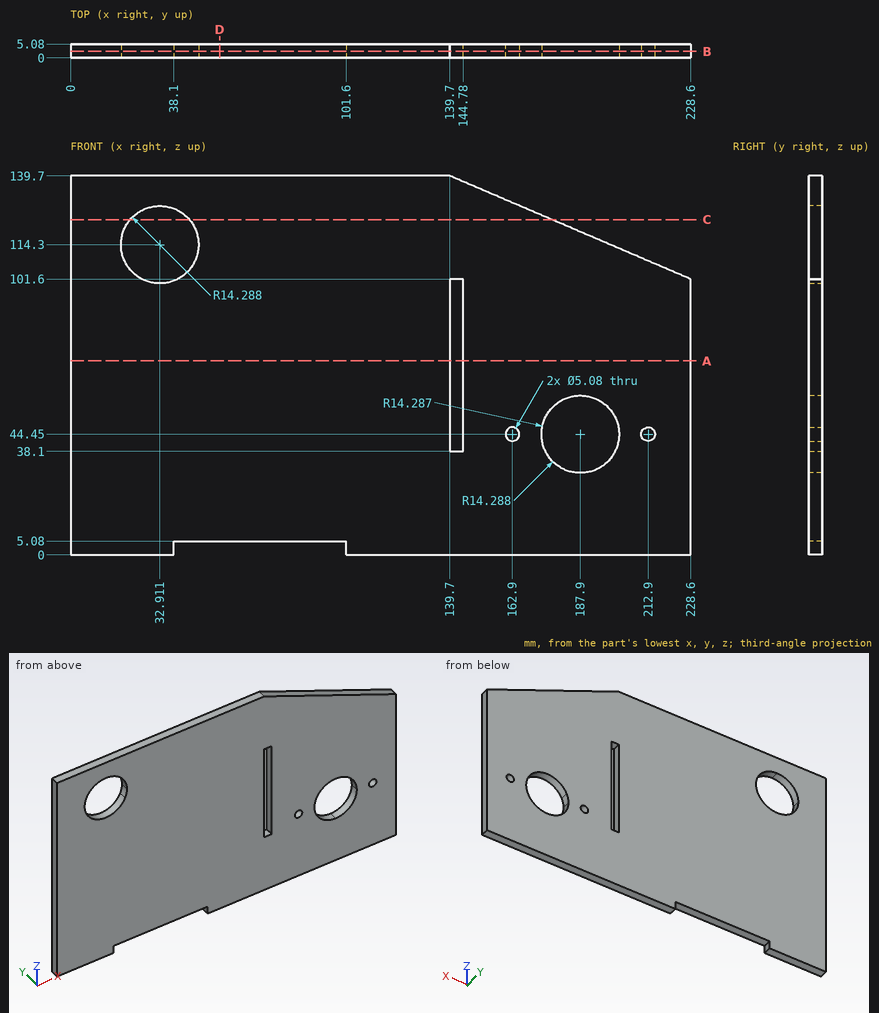
Part print with two shaded views. Sizes in mm from the minimum x, y, z corner. Give positions to 0.01 mm unless a question says otherwise; leave off trailing zeros. Order: outer loops, then holes, each group sorted by start corner. A loop starts at its lowest first (then second) coordinate and runs counter-clockwise, first axis right, second up.
1) Saw through at B-B, the plane y = 2.35. Count the separate pieces of the cut face and the enclosed holes in it, then the cut area to 3 significant figures.
2) Wall check: probe 1 along X at (y, z) = (4.45, 44.5); probe 2 along X at (y, z) = (0.3, 70); probe 3 along Z at (x, y) = (89, 4.55). Give the ranges that are in metal, low to high.
3) Saw through at A-A, the plane z = 71.5. Write the cut outline in (x, y).
4) Saw through at C-C, the plane z = 123.5. Write the cut outline in (x, y).
5) Saw through at D-D, the plane x = 55. Write the cut outline in (y, z).
Computed:
1. separate pieces: 1
1. enclosed holes: 5
1. area: 28,300 mm2
2. probe 1: x = 0 to 139.7, 144.78 to 160.36, 165.44 to 173.61, 202.19 to 210.36, 215.44 to 228.6
2. probe 2: x = 0 to 139.7, 144.78 to 228.6
2. probe 3: z = 5.08 to 139.7
3. outline: (0, 0) - (139.7, 0) - (139.7, 5.08) - (0, 5.08) - close; (144.78, 0) - (228.6, 0) - (228.6, 5.08) - (144.78, 5.08) - close
4. outline: (0, 0) - (21.98, 0) - (21.98, 5.08) - (0, 5.08) - close; (43.84, 0) - (177.5, 0) - (177.5, 5.08) - (43.84, 5.08) - close
5. outline: (0, 5.08) - (5.08, 5.08) - (5.08, 139.7) - (0, 139.7) - close
